from build123d import *

# Parameters (mm, degrees)
BOSS_EXTRUDE1_DEPTH = 12.5
SKETCH2_R           = 3
SKETCH2_R_2         = 6.25
BOSS_EXTRUDE2_DEPTH = 4.5
SKETCH3_R           = 2.5
SKETCH3_R_2         = 1
BOSS_EXTRUDE3_DEPTH = 3
SKETCH4_R           = 1
CUT_EXTRUDE1_DEPTH  = 2
FILLET1_R           = 2
CHAMFER1_SIZE       = 5
CHAMFER1_SIZE2      = 1.528653407


with BuildPart() as part:
    # Sketch1 → Boss-Extrude1 (new body)
    with BuildSketch(Plane(origin=(0, 0, 0), x_dir=(1, 0, 0), z_dir=(0, 1, 0))):
        Polygon((-12, 0), (-12, 16), (-16.5, 16), (-16.5, 18), (-12, 18), (-12, 22), (12, 22), (12, 18), (16.5, 18), (16.5, 16), (12, 16), (12, 0), align=None)
    extrude(amount=BOSS_EXTRUDE1_DEPTH)

    # Sketch2 → Boss-Extrude2 (add)
    with BuildSketch(Plane(origin=(0, 0, -22), x_dir=(-1, 0, 0), z_dir=(0, 0, -1))):
        with Locations((0.48292805, 6.25)):
            Circle(SKETCH2_R)
        with Locations((-5, 6.25)):
            Circle(SKETCH2_R_2)
    extrude(amount=BOSS_EXTRUDE2_DEPTH)

    # Sketch3 → Boss-Extrude3 (add)
    with BuildSketch(Plane(origin=(0, 0, -26.5), x_dir=(-1, 0, 0), z_dir=(0, 0, -1))):
        with Locations((-5, 6.25)):
            Circle(SKETCH3_R)
        with Locations((-5, 6.25)):
            Circle(SKETCH3_R_2, mode=Mode.SUBTRACT)
    extrude(amount=BOSS_EXTRUDE3_DEPTH)

    # Sketch4 → Cut-Extrude1 (cut)
    with BuildSketch(Plane(origin=(0, 0, -18), x_dir=(-1, 0, 0), z_dir=(0, 0, -1))):
        with Locations((-14.5, 6.25)):
            Circle(SKETCH4_R)
        with Locations((-14.5, 10.25)):
            Circle(SKETCH4_R)
        with Locations((-14.5, 2.25)):
            Circle(SKETCH4_R)
    cut_extrude1 = extrude(amount=-CUT_EXTRUDE1_DEPTH, mode=Mode.SUBTRACT)

    # Mirror1: Cut-Extrude1 across plane
    add(cut_extrude1.mirror(Plane(origin=(0, 0, 0), x_dir=(0, 0, 1), z_dir=(1, 0, 0))), mode=Mode.SUBTRACT)

    # Fillet1
    fillet1_edges = [part.edges().sort_by_distance(p)[0] for p in [
        (-16.5, 0, -17),
        (16.5, 12.5, -17),
        (16.5, 0, -17),
        (-16.5, 12.5, -17),
    ]]
    fillet(fillet1_edges, radius=FILLET1_R)

    # Chamfer1
    chamfer1_edges = [part.edges().sort_by_distance(p)[0] for p in [
        (-12, 6.25, -22),
    ]]
    chamfer1_side = [part.faces().sort_by_distance(p)[0] for p in [
        (-6.176633795, 6.25, -22),
    ]]
    chamfer(chamfer1_edges, length=CHAMFER1_SIZE, length2=CHAMFER1_SIZE2, reference=chamfer1_side[0])


solid = part.part
Work out the finished part from the listing and answer in its coordinate system (mm). A direction names the side the tool comes from. Give positions to 0.01 mm unless a question says otherwise; leave off trailing zeros. Loops run counter-clockwise (first coordinate to the right, second up) from the corner with the lowest first, then second, coordinate; pieces in that order, holes last. Notation, with made-up numbers: (64, -38.75) - (69, -38.75) arc R23 ccw to (69, -2.75) - close; hole circle Ø8 at (-9, -12.5). An arc over 180 degrees is marked (long way). Answer in a Markdown table with one row per item. Add a question column.
Q1. Consider line 1 along Y through (x, z) = (14.5, -17.45); line 2 along X through (y, z) = (6.75, -16.25); line 3 along Y through (x, z) = (5, -28.6). Determine where each line is inside the solid, lowest interval first.
Q2. The part is cut by section A-A (x = 10). Determine the outline of the cut face in (y, z).
Q3. Each of these flat-tipped pins is pushed along its axis until it touches: P1, Ø1.2, axis at x = 14.5, y = 2.25, coming from the +Z side; P2, Ø3.5, axis at x = 14.5, y = 7.5, coming from the +Z side; P3, Ø6, axis at x = -0.5, y = 4.5, coming from the -Z side; P4, Ø3, axis at x = 14.5, y = 6.25, coming from the -Z side. Where does it stop, or does it pass through?
Q4. The part is cut by section B-B (z = -9.25). Determine the outline of the cut face in (x, y), and give its area (3 significant figures).
Q5. Determine the mould class of faces 4 (the cylindrical face through (-15.9, 0.57, -17.01)), 5 (the flat face through (-13, 6, -16)), 6 (the cylindrical face through (-13.546, 6.55, -17.014)), 7 (the flat face through (5, 6, -26.5)) for opening direction Y: released by +Y, released by -Y, zero draft, split by the parting line, or undercut.
Q6. A tool of negligible diameter and unlimited length cuts with its end or side. For faces 1 (the flat face through (13, 6, -16)), 2 (the cylindrical face through (2.615, 7.001, -27.979)), 3 (the flat face through (12, 6, -20)), from which of +Z, -Z, +X, -X, +Y, -Y can it reach the whole face along a straight path? Write none if from no direction.
Q7. The part is cut by section D-D (z = -25.25). Determine the outline of the cut face in (x, y), and give its area (3 significant figures).
Solution:
| question | item | result |
|---|---|---|
| 1 | line 1 | y = 0 to 1.25, 3.25 to 5.25, 7.25 to 9.25, 11.25 to 12.5 |
| 1 | line 2 | x = -16.5 to -15.37, -13.63 to 13.63, 15.37 to 16.5 |
| 1 | line 3 | y = 3.75 to 5.25, 7.25 to 8.75 |
| 2 | outline | (0, -22) - (2.5, -22) - (2.5, -26.5) - (10, -26.5) - (10, -22) - (12.5, -22) - (12.5, 0) - (0, 0) - close |
| 3 | P1 | passes through |
| 3 | P2 | stops at z = -16 |
| 3 | P3 | stops at z = -26.5 |
| 3 | P4 | stops at z = -18 |
| 4 | outline | (-12, 0) - (12, 0) - (12, 12.5) - (-12, 12.5) - close |
| 4 | area | 300 mm² |
| 5 | face 4 | released by -Y |
| 5 | face 5 | zero draft |
| 5 | face 6 | undercut |
| 5 | face 7 | undercut |
| 6 | face 1 | +Z, +X, +Y, -Y |
| 6 | face 2 | -Z |
| 6 | face 3 | -Z, +X, +Y, -Y |
| 7 | outline | (-0.48, 3.25) arc R6.25 ccw (long way) to (-0.48, 9.25) arc R3 ccw to start |
| 7 | area | 134 mm² |
